from build123d import *

# Parameters (mm, degrees)
F0_W      = 154.4681414962
F0_H      = 32.4599891901
F1_DEPTH  = 48.0146426708
F2_W      = 11.2775340676
F2_H      = 24.0073213354
F3_DEPTH  = 154.6795647591
F4_W      = 20.4018931836
F4_H      = 24.0073213354
F4_W_2    = 3.5617277026
F4_W_3    = 3.5835206509
F4_W_4    = 3.6845356226
F4_W_5    = 4.9127191305
F4_W_6    = 22.562906146
F4_H_2    = 23.4004920349
F5_DEPTH  = 11.8805598468
F7_DEPTH  = 10.7736643404
F9_DEPTH  = 20.0494788587
F11_DEPTH = 21.1268346757
F12_W     = 1.8992722034
F12_H     = 24.0073213354
F13_DEPTH = 13.5909728706


with BuildPart() as f1:
    # F0 (on Top) → F1 (new body)
    with BuildSketch(Plane.XY):
        with Locations((3.7253e-06, -0.5876496434)):
            Rectangle(F0_W, F0_H)
    extrude(amount=F1_DEPTH)

    # F2 (on face) → F3 (join)
    with BuildSketch(Plane.YZ.offset(77.2340744734)):
        with Locations((-22.4564112723, 36.0109820031)):
            Rectangle(F2_W, F2_H)
        Polygon((-16.8176442385, 13.3598086642), (-16.8176442385, 24.0073213354), (-28.0951783061, 24.0073213354), align=None)
    extrude(amount=-F3_DEPTH)

    # F4 (on face) → F5 (cut)
    with BuildSketch(Plane.XZ.offset(28.0951783061)):
        with Locations((-67.244543694, 12.0036606677)):
            Rectangle(F4_W, F4_H)
        with Locations((-67.244543694, 36.0109820031)):
            Rectangle(F4_W, F4_H)
        with Locations((-36.5212969482, 12.0036606677)):
            Rectangle(F4_W_2, F4_H)
        with Locations((-36.5212969482, 36.0109820031)):
            Rectangle(F4_W_2, F4_H)
        with Locations((-17.2269493341, 36.0109820031)):
            Rectangle(F4_W_3, F4_H)
        with Locations((-17.2269493341, 12.0036606677)):
            Rectangle(F4_W_3, F4_H)
        with Locations((19.1767290235, 36.0109820031)):
            Rectangle(F4_W_4, F4_H)
        with Locations((19.1767290235, 12.0036606677)):
            Rectangle(F4_W_4, F4_H)
        with Locations((38.9504507184, 12.0036606677)):
            Rectangle(F4_W_5, F4_H)
        with Locations((65.9526214004, 36.0109820031)):
            Rectangle(F4_W_6, F4_H)
        with Locations((65.9526214004, 12.0036606677)):
            Rectangle(F4_W_6, F4_H)
        with Locations((38.9504507184, 35.7075673528)):
            Rectangle(F4_W_5, F4_H_2)
    extrude(amount=-F5_DEPTH, mode=Mode.SUBTRACT)

    # F6 (on face) → F7 (join)
    with BuildSketch(Plane.XY.offset(48.0146426708)):
        Polygon((-57.0435971022, -16.2146184593), (-77.2340670228, -16.2146184593), (-77.2340670228, -43.9355224371), (-57.0435971022, -43.9355224371), (-57.0435971022, -28.0951783061), align=None)
        with BuildLine():
            Line((-57.0435971022, -43.9355224371), (-77.2340670228, -43.9355224371))
            ThreePointArc((-77.2340670228, -43.9355224371), (-67.1388320625, -54.0307573974), (-57.0435971022, -43.9355224371))
        make_face()
        Polygon((77.2340744734, -43.4713661671), (77.2340744734, -16.2146184593), (54.6711683273, -16.2146184593), (54.6711683273, -28.0951783061), (54.6711683273, -43.4713661671), align=None)
        with BuildLine():
            ThreePointArc((54.6711683273, -43.4713661671), (65.9526214004, -54.7528192401), (77.2340744734, -43.4713661671))
            Line((77.2340744734, -43.4713661671), (54.6711683273, -43.4713661671))
        make_face()
    extrude(amount=-F7_DEPTH)

    # F8 (on face) → F9 (join)
    with BuildSketch(Plane(origin=(-77.2340670228, 0, 0), x_dir=(0, -1, 0), z_dir=(-1, 0, 0))):
        Polygon((30.0750704482, 18.6204891652), (43.9355224371, 37.2409783304), (16.2146184593, 37.2409783304), (16.2146184593, 18.6204891652), (23.1448444538, 18.6204891652), align=None)
        Polygon((16.2146184593, 9.3102445826), (23.1448444538, 18.6204891652), (16.2146184593, 18.6204891652), align=None)
    extrude(amount=-F9_DEPTH)

    # F10 (on face) → F11 (join)
    with BuildSketch(Plane.YZ.offset(77.2340744734)):
        Polygon((-16.2146184593, 37.2409783304), (-43.4713661671, 37.2409783304), (-30.2190445364, 19.3241238594), (-23.1028571725, 19.3241238594), (-16.2146184593, 8.6756854873), align=None)
    extrude(amount=-F11_DEPTH)

    # F12 (on face) → F13 (cut)
    with BuildSketch(Plane.XZ.offset(28.0951783061)):
        with Locations((0.9496361017, 36.0109820031)):
            Rectangle(F12_W, F12_H)
        with Locations((0.9496361017, 12.0036606677)):
            Rectangle(F12_W, F12_H)
    extrude(amount=-F13_DEPTH, mode=Mode.SUBTRACT)


solid = f1.part
Work out the finished part from the listing and answer in its coordinate system (mm). A direction names the side the tool comes from. Coordinates: 2 decimals unless noted, no trailing zeros. Order: outer loops, then holes, each group sorted by start corner. A loop starts at its lowest first (then second) coordinate and runs counter-clockwise, first axis right, second up. Notation, with made-up numbers: (75, 24.5) - (119, 24.5) arc R25 ccw to (119, 59.5) - close; hole circle Ø9 at (84, 55). An arc over 180 degrees is marked (long way). Put each result on its own line as item: value. Start each with the question number.
1) For faces 1 (the flat face through (-67, -27, 18.62)), 2 (the flat face through (-47.54, -22.54, 18.76)), 3 (the flat face through (10, -28.095, 36)), determine the directions among +Z, -Z, +X, -X, +Y, -Y from which every point of the face is accessible in a straight line to the end or side of a thin tool.
2) Find section A-A (z = 44). Give the vertices of the cut face in (x, y), plus the area to 3 significant figures.
3) Find section C-C (y = -26.5). State how many separate pieces and enclosed holes the cut face has, plus the area to 3 significant figures.
4) For a pull along X with two mould halves and no side action, classify faces 4 (the flat face through (-1, -11, 48.015)), 5 (the flat face through (0, -21, 30)), 6 (the flat face through (-17, -16.215, 24)) as released by +X, released by -X, zero draft, split by the parting line, or undercut.
5) Flat-ended cylindrical pins translate along their axes: pin 1 (7 mm diameter, centred on x = 69.5, y = -41.5, fed in from -Z); pin 2 (1.5 mm diameter, centred on x = 39.5, z = 15, fed in from -Y); pin 3 (4 mm diameter, centred on x = -18, z = 17.5, fed in from -Y). Find the tip coordinate at first contact, or state that the pin passes through.
6) Find the intervals of material crossed by line 1 (X direction, y = -15.5, z = 19.5); line 2 (X direction, y = -39.5, z = 41); line 3 (Y direction, x = -4.5, z = 28.5), in increasing order. Write a range as from..to.
7) Find section D-D (y = -36). Give the vertices of the cut face in (x, z).
8) Find section B-B (x = 3.5). Give the vertices of the cut face in (y, z).
Results list:
1. face 1: -Z, +X, -X, -Y
1. face 2: -Z, -Y
1. face 3: +Z, -Z, -Y
2. outline: (-77.23, -43.94) arc R10.1 ccw to (-57.04, -43.94) - (-57.04, -28.1) - (-38.3, -28.1) - (-38.3, -16.21) - (-34.74, -16.21) - (-34.74, -28.1) - (-19.02, -28.1) - (-19.02, -16.21) - (-15.44, -16.21) - (-15.44, -28.1) - (0, -28.1) - (0, -14.5) - (1.9, -14.5) - (1.9, -28.1) - (17.33, -28.1) - (17.33, -16.21) - (21.02, -16.21) - (21.02, -28.1) - (36.49, -28.1) - (36.49, -16.21) - (41.41, -16.21) - (41.41, -28.1) - (54.67, -28.1) - (54.67, -43.47) arc R11.28 ccw to (77.23, -43.47) - (77.23, 15.64) - (-77.23, 15.64) - close
2. area: 7,570 mm^2
3. separate pieces: 5
3. enclosed holes: 0
3. area: 3,620 mm^2
4. face 4: zero draft
4. face 5: undercut
4. face 6: undercut
5. pin 1: stops at z = 29.84
5. pin 2: stops at y = -16.21
5. pin 3: stops at y = -23.03
6. line 1: x = -77.23..0, 1.9..77.23
6. line 2: x = -77.23..-57.04, 54.67..77.23
6. line 3: y = -28.1..15.64
7. outline: (-77.23, 26.58) - (-57.18, 26.58) - (-57.18, 37.24) - (-57.04, 37.24) - (-57.04, 48.01) - (-77.23, 48.01) - close; (54.67, 37.24) - (56.11, 37.24) - (56.11, 27.14) - (77.23, 27.14) - (77.23, 48.01) - (54.67, 48.01) - close
8. outline: (-28.1, 24.01) - (-16.82, 13.36) - (-16.82, 0) - (15.64, 0) - (15.64, 48.01) - (-28.1, 48.01) - close
